Autodesk Inventor part; units mm, degrees
ref_plane "YZ Plane" through (0, 0, 0) normal (1, 0, 0) x (0, 1, 0)
ref_plane "XZ Plane" through (0, 0, 0) normal (0, 1, 0) x (-1, 0, 0)
ref_plane "XY Plane" through (0, 0, 0) normal (0, 0, 1) x (1, 0, 0)
sketch "Sketch1" plane through (0, 0, 0) normal (0, 0, 1) x (1, 0, 0)
  circle A0 centre (0, 0) radius 4
  arc A1 (-0.7484, 5.6809) -> (0.7484, 5.6809) centre (0, 5.73) ccw
  arc A2 (-3.4886, 4.5456) -> (-2.1923, 5.294) centre (-2.865, 4.9623) ccw
  arc A3 (-5.294, 2.1923) -> (-4.5456, 3.4886) centre (-4.9623, 2.865) ccw
  arc A4 (-5.6809, -0.7484) -> (-5.6809, 0.7484) centre (-5.73, 0) ccw
  arc A5 (-4.5456, -3.4886) -> (-5.294, -2.1923) centre (-4.9623, -2.865) ccw
  arc A6 (-2.1923, -5.294) -> (-3.4886, -4.5456) centre (-2.865, -4.9623) ccw
  arc A7 (0.7484, -5.6809) -> (-0.7484, -5.6809) centre (0, -5.73) ccw
  arc A8 (3.4886, -4.5456) -> (2.1923, -5.294) centre (2.865, -4.9623) ccw
  arc A9 (5.294, -2.1923) -> (4.5456, -3.4886) centre (4.9623, -2.865) ccw
  arc A10 (5.6809, 0.7484) -> (5.6809, -0.7484) centre (5.73, 0) ccw
  arc A11 (4.5456, 3.4886) -> (5.294, 2.1923) centre (4.9623, 2.865) ccw
  arc A12 (2.1923, 5.294) -> (3.4886, 4.5456) centre (2.865, 4.9623) ccw
  arc A13 (-0.7484, 5.6809) -> (-2.1923, 5.294) centre (0, 0) ccw
  arc A14 (-3.4886, 4.5456) -> (-4.5456, 3.4886) centre (0, 0) ccw
  arc A15 (-5.294, 2.1923) -> (-5.6809, 0.7484) centre (0, 0) ccw
  arc A16 (-5.6809, -0.7484) -> (-5.294, -2.1923) centre (0, 0) ccw
  arc A17 (2.1923, 5.294) -> (0.7484, 5.6809) centre (0, 0) ccw
  arc A18 (4.5456, 3.4886) -> (3.4886, 4.5456) centre (0, 0) ccw
  arc A19 (5.6809, 0.7484) -> (5.294, 2.1923) centre (0, 0) ccw
  arc A20 (5.294, -2.1923) -> (5.6809, -0.7484) centre (0, 0) ccw
  arc A21 (3.4886, -4.5456) -> (4.5456, -3.4886) centre (0, 0) ccw
  arc A22 (0.7484, -5.6809) -> (2.1923, -5.294) centre (0, 0) ccw
  arc A23 (-4.5456, -3.4886) -> (-3.4886, -4.5456) centre (0, 0) ccw
  arc A24 (-2.1923, -5.294) -> (-0.7484, -5.6809) centre (0, 0) ccw
  dimension "d0" = 8
  dimension "d2" = 1.5
  dimension "d5" = 360
extrude "Extrusion1" add sketch "Sketch1" along normal blind 9
properties part number "poulie 12 dents"
Check sheet for the modelled part. Datum: model origin and axes. Units: mm. Give positions to 0.01 mm unless a question says otherwise; leave off trailing zeros. Loops run counter-clockwise (first coordinate to the right, second up) from the corner with the lowest first, then second, coordinate; pieces in that order, holes last. Notation, with made-up numbers: M 15,46 L 47,46 A17 cw 47,72 Z; hole C 69.5,47.5 d8. An arc over 180 degrees is marked long. Return JSON: item names as keys, results as strings. Group by question number.
1. Mould release check, pull along Y, two halves, no side actions. Record for faces 1 (the cylindrical face through (1.47, 5.54, 4.44)), 2 (the cylindrical face through (4.32, 2.48, 4.44)), 3 (the cylindrical face through (-0.02, -4.98, 4.44)): released by +Y, released by -Y, zero draft, split by the parting line, or undercut.
2. Cross-section at A-A on x = 0. Record the boundary of the cut face in (y, z).
3. Go/stop test with a flat-tipped pin: pin 1 (5 mm diameter, centred on x = 0, y = 0, fed in from -Z). Record where the tip stops, or that it passes through.
4. Cross-section at C-C on z = 2.5. Record the boundary of the cut face in (x, y) (3 decimals).
5. Thickness scan on L1, parallel to Y at x = 0, z = 3.5; L2, parallel to Y at x = -2.75, z = 0.5; L3, parallel to X at y = -2, z = 3.25. Record the ranges inside material, lowest first.
Return value:
{
 "1": {"face 1": "released by +Y", "face 2": "undercut", "face 3": "released by -Y"},
 "2": {"outline": "M -4.98,0 L -4,0 L -4,9 L -4.98,9 Z; M 4,0 L 4.98,0 L 4.98,9 L 4,9 Z"},
 "3": {"pin 1": "through"},
 "4": {"outline": "M -5.681,-0.748 A5.729 ccw -5.294,-2.192 A0.75 cw -4.546,-3.489 A5.73 ccw -3.489,-4.546 A0.75 cw -2.192,-5.294 A5.731 ccw -0.748,-5.681 A0.75 cw 0.748,-5.681 A5.729 ccw 2.192,-5.294 A0.75 cw 3.489,-4.546 A5.73 ccw 4.546,-3.489 A0.75 cw 5.294,-2.192 A5.731 ccw 5.681,-0.748 A0.75 cw 5.681,0.748 A5.729 ccw 5.294,2.192 A0.75 cw 4.546,3.489 A5.73 ccw 3.489,4.546 A0.75 cw 2.192,5.294 A5.731 ccw 0.748,5.681 A0.75 cw -0.748,5.681 A5.729 ccw -2.192,5.294 A0.75 cw -3.489,4.546 A5.73 ccw -4.546,3.489 A0.75 cw -5.294,2.192 A5.731 ccw -5.681,0.748 A0.75 cw Z; hole C 0,0 d8"},
 "5": {"L1": "-4.98 to -4, 4 to 4.98", "L2": "-4.22 to -2.9, 2.9 to 4.22", "L3": "-5.37 to -3.46, 3.46 to 5.37"}
}
